Can you work these out from the drawing? Everything is in mm from the part's minimum corner. A direction names the side the tool comes from. Coordinates: 2 decimals unless noted, no trailing zeros. Order: outer loops, then holes, each group sorted by start corner. A loop starts at its lowest first (then second) coordinate and runs counter-clockwise, first axis right, second up. Notation, with made-up numbers: (61.5, 60) -> (70.5, 60) arc R14 ccw to (70.5, 82) -> close; hole circle Ø7 at (1.5, 39). An arc over 180 degrees is marked (long way). Put each result on its own line as item: value. Start each with the question number.
Q1. Will these pins go through, and if not, where does the flat tip stop? pin 1 (1.5 mm diameter, centred on x = 43.5, y = 63.5, fed in from -Z); pin 2 (18 mm diameter, centred on x = 9.5, y = 72, fed in from +Z); pin 3 (8 mm diameter, centred on x = 86, z = 47, fed in from -Y); pin 4 (15 mm diameter, centred on y = 30, z = 89, fed in from -X).
Q2. If we section it at C-C (y = 32): Please give me the cut outline in (x, z).
Q3. For the marked faces 1, 2, 3 and 4, which set-ups out of +Z, -Z, +X, -X, +Y, -Y let a thin tool reach every point of the face, with its end or its side?
Q4. If we section it at D-D (z = 62.5): Please give me the cut outline in (x, y), and give its area (3 significant figures).
Q5. If we section it at B-B (x = 92.5): Please give me the cut outline in (y, z).
Q6. If we section it at A-A (z = 21.5): Please give me the cut outline in (x, y), and give its area (3 significant figures).
Q7. Please list where these lines run through material, in increasing order: line 1 along X through (y, z) = (54.5, 16); line 2 along X through (y, z) = (92, 86.5); line 3 along Z through (x, y) = (42, 67.5).
Q8. We'd pull the mould along X, two halves only. Please class the marked faces 5, 6, 7 and 8: +X half, -X half, draft (parallel to the pull), parting line (faces both ways), or undercut.
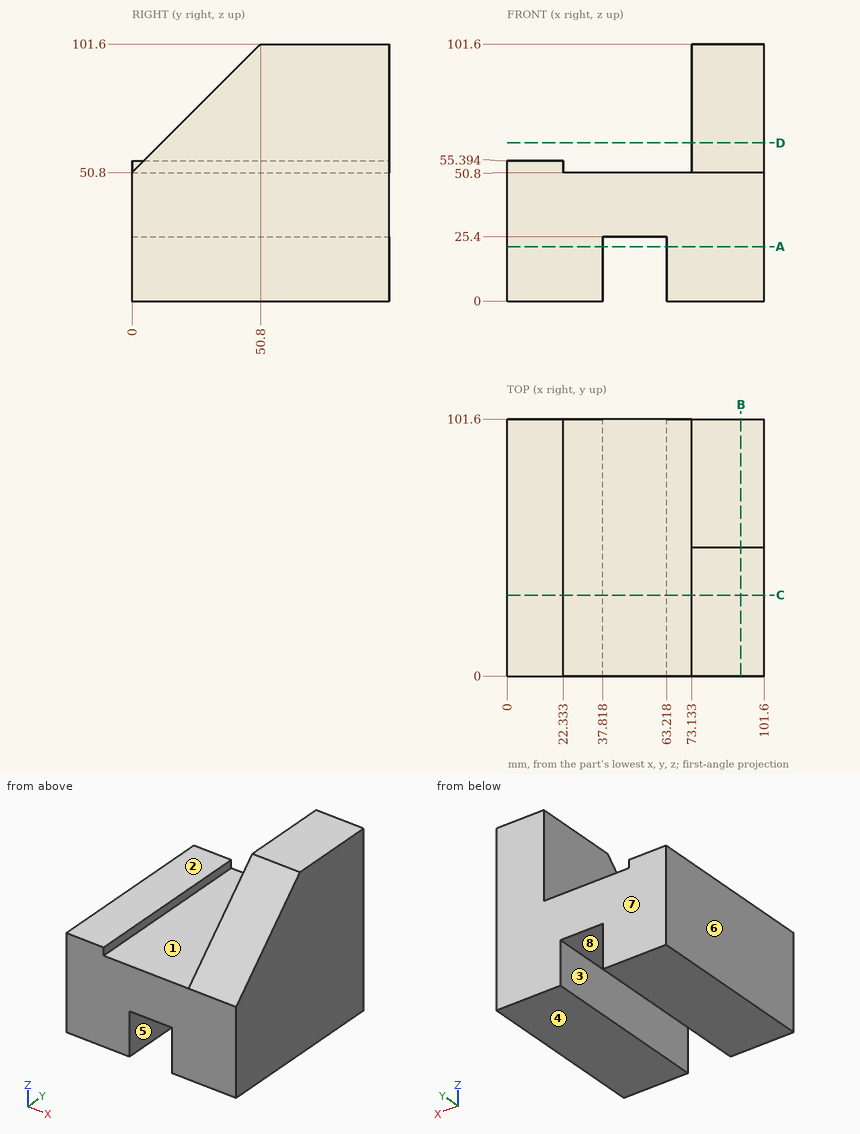
The answers:
1. pin 1: z = 25.4
1. pin 2: z = 55.39
1. pin 3: y = 0
1. pin 4: x = 73.13
2. outline: (0, 0) -> (37.82, 0) -> (37.82, 25.4) -> (63.22, 25.4) -> (63.22, 0) -> (101.6, 0) -> (101.6, 82.8) -> (73.13, 82.8) -> (73.13, 50.8) -> (22.33, 50.8) -> (22.33, 55.39) -> (0, 55.39) -> close
3. face 1: +Z, +Y, -Y
3. face 2: +Z, -X, +Y, -Y
3. face 3: -Z, +Y, -Y
3. face 4: -Z, +X, -X, +Y, -Y
4. outline: (73.13, 11.7) -> (101.6, 11.7) -> (101.6, 101.6) -> (73.13, 101.6) -> close
4. area: 2,560 mm^2
5. outline: (0, 0) -> (101.6, 0) -> (101.6, 101.6) -> (50.8, 101.6) -> (0, 50.8) -> close
6. outline: (0, 0) -> (37.82, 0) -> (37.82, 101.6) -> (0, 101.6) -> close; (63.22, 0) -> (101.6, 0) -> (101.6, 101.6) -> (63.22, 101.6) -> close
6. area: 7,740 mm^2
7. line 1: 0 to 37.82, 63.22 to 101.6
7. line 2: 73.13 to 101.6
7. line 3: 25.4 to 50.8
8. face 5: undercut
8. face 6: -X half
8. face 7: draft
8. face 8: undercut
